Work out the finished part from the listing and answer in its coordinate system (mm). A direction names the side the tool comes from. Round coordinates to 2 decimals unless told otherwise and drop trailing zeros. Loops run counter-clockwise (first coordinate to the right, second up) from the corner with the lowest first, then second, coordinate; pieces in that order, holes last. Notation, with made-up numbers: (26.25, 18.25) - (41.25, 18.25) arc R14 cw to (41.25, 34.25) - close; hole circle Ø11 at (-12.75, -4). An arc over 180 degrees is marked (long way). Answer as CSV lines item,"result". Start each with the question number.
Q1. Section B-B on y = -13 is taken. Write down the section's boundary in (x, z).
Q2. Each of these flat-tipped pins is pushed along its axis until it touches: pin 1 Ø3 at (y, z) = (8.5, -3) entering from -X; pin 2 Ø11 at (x, y) = (-2, 2) entering from -Z (3 decimals); pin 3 Ø3 at (x, y) = (-3.5, 9.5) entering from -Z; pin 4 Ø1 at (y, z) = (-3.5, -4.5) entering from -X. Where does it stop, or does it pass through?
Q3. For faces 4 (the face through (17.223, 10.13, -2.74)), 5 (the face through (-18.95, -11.14, -2.74)), 6 (the face through (-19.125, 10.837, -2.74)), determine the directions among +Z, -Z, +X, -X, +Y, -Y from which every point of the face is accessible in a straight line to the end or side of a thin tool.
Q4. Section A-A on x = 0 is taken. Write down the section's boundary in (y, z) (3 decimals).
Q5. The mould has two halves that part along Y. Classify faces 1 (the face through (19, 8, -3.5)), 2 (the face through (18.95, 11.14, -2.74)), 3 (the face through (0, -19.981, -3)): +Y half, -Y half, draft (parallel to the pull), parting line (faces both ways), or undercut.
Q6. Straight lines are drawn through the part: L1, parallel to Y at x = 0, z = -2.65; L2, parallel to Y at x = 0, z = -3.85; L3, parallel to Y at x = 0, z = -2.9. For each, find the intervals that lie inside material, in ascending order. Write a range as [from, to].
```python
from build123d import *

# Parameters (mm, degrees)
PAD_DEPTH     = 2
SKETCH001_R   = 8
SKETCH001_R_2 = 5.08
PAD001_DEPTH  = 3.175
FILLET_R      = 2
PAD002_DEPTH  = 1.5


with BuildPart() as part:
    # Sketch → Pad (new body)
    with BuildSketch(Plane(origin=(0, 0, 0), x_dir=(1, 0, 0), z_dir=(0, 0, -1))):
        Polygon((30, 0), (15, 25.980762), (-15, 25.980762), (-30, 0), (-15, -25.980762), (15, -25.980762), align=None)
    extrude(amount=PAD_DEPTH)

    # Sketch001 → Pad001 (new body)
    with BuildSketch(Plane(origin=(0, 0, -2), x_dir=(1, 0, 0), z_dir=(0, 0, -1))):
        Circle(SKETCH001_R)
        Circle(SKETCH001_R_2, mode=Mode.SUBTRACT)
    extrude(amount=PAD001_DEPTH)

    # Fillet
    fillet_edges = [part.edges().sort_by_distance(p)[0] for p in [
        (-8, 0, -2),
    ]]
    fillet(fillet_edges, radius=FILLET_R)

    # Sketch002 → Pad002 (new body)
    with BuildSketch(Plane(origin=(0, 0, -2), x_dir=(1, 0, 0), z_dir=(0, 0, -1))):
        Polygon((12.690599, -21.980762), (25.381198, 0), (12.690599, 21.980762), (-12.690599, 21.980762), (-25.381198, 0), (-12.690599, -21.980762), align=None)
        Polygon((11.535898, -19.980762), (23.071797, 0), (11.535898, 19.980762), (-11.535898, 19.980762), (-23.071797, 0), (-11.535898, -19.980762), align=None, mode=Mode.SUBTRACT)
    extrude(amount=PAD002_DEPTH)


solid = part.part
```
Findings:
1,outline,"(-22.49, -2) - (-17.88, -2) - (-17.88, -3.5) - (-15.57, -3.5) - (-15.57, -2) - (15.57, -2) - (15.57, -3.5) - (17.88, -3.5) - (17.88, -2) - (22.49, -2) - (22.49, 0) - (-22.49, 0) - close"
2,pin 1,"stops at x = -25.74"
2,pin 2,"stops at z = -5.175"
2,pin 3,"stops at z = -2.55"
2,pin 4,"stops at x = -7.42"
3,face 4,"-Z"
3,face 5,"-Z, -X, -Y"
3,face 6,"-Z, -X, +Y"
4,outline,"(-25.981, -2) - (-21.981, -2) - (-21.981, -3.5) - (-19.981, -3.5) - (-19.981, -2) - (-10, -2) arc R2 cw to (-8, -4) - (-8, -5.175) - (-5.08, -5.175) - (-5.08, -2) - (5.08, -2) - (5.08, -5.175) - (8, -5.175) - (8, -4) arc R2 cw to (10, -2) - (19.981, -2) - (19.981, -3.5) - (21.981, -3.5) - (21.981, -2) - (25.981, -2) - (25.981, 0) - (-25.981, 0) - close"
5,face 1,"draft"
5,face 2,"+Y half"
5,face 3,"undercut"
6,L1,"y = [-21.98, -19.98], [-8.52, -5.08], [5.08, 8.52], [19.98, 21.98]"
6,L2,"y = [-8.01, -5.08], [5.08, 8.01]"
6,L3,"y = [-21.98, -19.98], [-8.33, -5.08], [5.08, 8.33], [19.98, 21.98]"
